The listing builds one solid part. Answer for the finished solid, in the listing's coordinates (mm). Coordinates: 2 decimals unless noted, no trailing zeros. Order: outer loops, then holes, each group sorted by start corner. A loop starts at its lowest first (then second) coordinate and runs counter-clockwise, first axis right, second up. Notation, with made-up numbers: (-28, 84) -> (2, 84) arc R19 ccw to (2, 106) -> close; hole circle Ø4 at (-11, 77.25). An arc over 180 degrees is marked (long way). Answer in a Markdown table with one row per item. Add a question column.
```python
from build123d import *

# Parameters (mm, degrees)
F1_DEPTH = 38.1


with BuildPart() as f1:
    # F0 (on Top) → F1 (new body)
    with BuildSketch(Plane.XY):
        with BuildLine():
            ThreePointArc((0, -22.908895), (-14.689808, -58.373229), (20.774525, -43.683421))
            ThreePointArc((20.774525, -43.683421), (14.689808, -28.993613), (0, -22.908895))
        make_face()
    extrude(amount=F1_DEPTH)

    # F4: sweep along a path in F2
    with BuildLine(Plane.XY) as f4_path:
        ThreePointArc((-72.136711, -192.550732), (-18.626108, -102.809884), (0, 0))
    # F3 (on Front) → F4 (sweep)
    with BuildSketch(Plane.XZ):
        with BuildLine():
            Line((-25.131127, 0), (25.131127, 0))
            ThreePointArc((25.131127, 0), (0, 25.131127), (-25.131127, 0))
        make_face()
    sweep(path=f4_path.line)

    # F5: sweep along a path in F2
    with BuildLine(Plane.XY) as f5_path:
        ThreePointArc((72.136711, -192.550732), (18.626108, -102.809884), (0, 0))
    # F4_face (on face) → F5 (sweep)
    with BuildSketch(Plane(origin=(0, 0, 10.665982), x_dir=(-1, 0, 0), z_dir=(0, 1, 0))):
        with BuildLine():
            Line((-25.131127, -10.665982), (25.131127, -10.665982))
            ThreePointArc((25.131127, -10.665982), (0, 14.465145), (-25.131127, -10.665982))
        make_face()
    sweep(path=f5_path.line)


solid = f1.part
```
Q1. A cutting plane is placed at B-B (z = 6). Determine the outline of the cut face in (x, y), then the cut area to 3 significant figures.
Q2. A cutting plane is placed at A-A (z = 32). Determine the outline of the cut face in (x, y).
Q3. Straight lines are drawn through the part: line 1 (X direction, y = -99.5, z = 22.5); line 2 (X direction, y = -189.5, z = 14); line 3 (Z direction, x = 11.5, y = -19). For each, find the intervals that lie inside material, in ascending order.
Q4. Given pin 1 (8 mm diameter, centred on x = -9.5, y = -108.5, fed in from +Z); pin 2 (12 mm diameter, centred on x = 26, y = -60.5, fed in from +Z); pin 3 (6 mm diameter, centred on y = -162, z = 24.5, fed in from -X), each flat-ended and moving along its own axis, determine where each tip first touches the part or whether it passes through.
Returned:
| question | item | result |
|---|---|---|
| 1 | outline | (-90.53, -176.52) -> (-53.74, -208.59) arc R317.46 ccw to (0, -122.06) arc R317.46 ccw to (53.74, -208.59) -> (90.53, -176.52) arc R268.65 cw to (24.4, 0) -> (-24.4, 0) arc R268.65 cw to start |
| 1 | area | 16,500 mm² |
| 2 | outline | circle Ø41.55 at (0, -43.68) |
| 3 | line 1 | x = -29.34 to -5.54, 5.54 to 29.34 |
| 3 | line 2 | x = -75.64 to -42.78, 42.78 to 75.64 |
| 3 | line 3 | z = 0 to 22.66 |
| 4 | pin 1 | stops at z = 24.26 |
| 4 | pin 2 | stops at z = 21.37 |
| 4 | pin 3 | stops at x = -64.99 |
